CAD build for the part. Positions are in the model's coordinates, mm. Face numbers are marked on the shaded views. A direction names the side the tool comes from. Coordinates: 2 decimals unless noted, no trailing zeros. Write each loop counter-clockwise with the first axis right and the second up, starting at its lowest first coordinate (ties: lowest second). Pieces come first, ordered by that corner, then holes. Notation, with made-up numbers: (73, 23) -> (117, 23) arc R19 ccw to (117, 28) -> close; hole circle Ø5 at (-35.5, 5.25). An arc over 180 degrees is marked (long way). Answer as CSV lines item,"result". Start each with the question number.
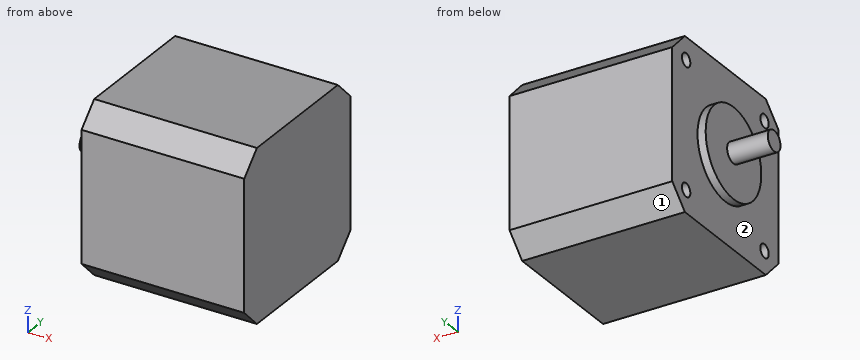
```python
from build123d import *

# Parameters (mm, degrees)
F0_W     = 42
F0_H     = 42
F0_R     = 1.65
F0_R_2   = 11
F0_R_3   = 2.5
F1_DEPTH = 40
F2_DEPTH = 2
F3_DEPTH = 12
F4_DEPTH = 10
F5_SIZE  = 5


with BuildPart() as f1:
    # F0 (on Right) → F1 (new body)
    with BuildSketch(Plane.YZ):
        Rectangle(F0_W, F0_H)
        with Locations((-15.5, -15.5)):
            Circle(F0_R, mode=Mode.SUBTRACT)
        with Locations((15.5, -15.5)):
            Circle(F0_R, mode=Mode.SUBTRACT)
        with Locations((-15.5, 15.5)):
            Circle(F0_R, mode=Mode.SUBTRACT)
        Circle(F0_R_2, mode=Mode.SUBTRACT)
        with Locations((15.5, 15.5)):
            Circle(F0_R, mode=Mode.SUBTRACT)
        with Locations((15.5, -15.5)):
            Circle(F0_R)
        with Locations((-15.5, -15.5)):
            Circle(F0_R)
        with Locations((-15.5, 15.5)):
            Circle(F0_R)
        with Locations((15.5, 15.5)):
            Circle(F0_R)
        Circle(F0_R_2)
        Circle(F0_R_3, mode=Mode.SUBTRACT)
        Circle(F0_R_3)
    extrude(amount=F1_DEPTH)

    # F0 (on Right) → F2 (join)
    with BuildSketch(Plane.YZ):
        Circle(F0_R_2)
        Circle(F0_R_3, mode=Mode.SUBTRACT)
        Circle(F0_R_3)
    extrude(amount=-F2_DEPTH)

    # F0 (on Right) → F3 (join)
    with BuildSketch(Plane.YZ):
        Circle(F0_R_3)
    extrude(amount=-F3_DEPTH)

    # F0 (on Right) → F4 (cut)
    with BuildSketch(Plane.YZ):
        with Locations((15.5, 15.5)):
            Circle(F0_R)
        with Locations((15.5, -15.5)):
            Circle(F0_R)
        with Locations((-15.5, 15.5)):
            Circle(F0_R)
        with Locations((-15.5, -15.5)):
            Circle(F0_R)
    extrude(amount=F4_DEPTH, mode=Mode.SUBTRACT)

    # F5
    f5_edges = [f1.edges().sort_by_distance(p)[0] for p in [
        (20, -21, 21),
        (20, 21, 21),
        (20, 21, -21),
        (20, -21, -21),
    ]]
    chamfer(f5_edges, length=F5_SIZE)


solid = f1.part
```
1. Tool access for the marked faces 1 and 2: list every direction of +Z, -Z, +X, -X, +Y, -Y with a clear straight run to the whole face (end or side of a thin tool).
2. Cut at B-B (z = 0). Give the cut face in (x, y).
3. Cut at D-D (x = 14). Give the cut face in (y, z).
4. Wall check: line 1 (Z direction, x = 5, y = -15.5); line 2 (X direction, y = 19, z = 13.5); line 3 (Y direction, x = 4, z = 15). Give the ranges that are in metal, low to high.
5. Cut at A-A (x = 5.5). Give the cut face in (y, z), then the cut area to 3 significant figures.
6. Flat gauge pins, fed straight in: P1, Ø6, axis at y = -15.5, z = 15, coming from the -X side; P2, Ø12, axis at y = 6.5, z = -7, coming from the -X side; P3, Ø1.6, axis at y = 16, z = 15, coming from the -X side. Where does each tip first touch, or does it go through?
Geometry check:
1,face 1,"-Z, +X, -X, +Y"
1,face 2,"-X"
2,outline,"(-12, -2.5) -> (-2, -2.5) -> (-2, -11) -> (0, -11) -> (0, -21) -> (40, -21) -> (40, 21) -> (0, 21) -> (0, 11) -> (-2, 11) -> (-2, 2.5) -> (-12, 2.5) -> close"
3,outline,"(-21, -16) -> (-16, -21) -> (16, -21) -> (21, -16) -> (21, 16) -> (16, 21) -> (-16, 21) -> (-21, 16) -> close"
4,line 1,"-21 to -17.15, -13.85 to 13.85, 17.15 to 21"
4,line 2,"0 to 40"
4,line 3,"-21 to -17.07, -13.93 to 13.93, 17.07 to 21"
5,outline,"(-21, -16) -> (-16, -21) -> (16, -21) -> (21, -16) -> (21, 16) -> (16, 21) -> (-16, 21) -> (-21, 16) -> close; hole circle Ø3.3 at (-15.5, -15.5); hole circle Ø3.3 at (-15.5, 15.5); hole circle Ø3.3 at (15.5, -15.5); hole circle Ø3.3 at (15.5, 15.5)"
5,area,"1,680 mm²"
6,P1,"x = 0"
6,P2,"x = -2"
6,P3,"x = 10"
